Source: CAD feature listing. Evaluate the final solid. Frame: model axes, mm. A direction names the side the tool comes from. Round coordinates to 2 decimals unless told otherwise and drop trailing zeros. Write each loop counter-clockwise with the first axis right and the second up, starting at its lowest first coordinate (ties: lowest second). Pieces come first, ordered by that corner, then holes. Notation, with made-up numbers: M -15,-15.5 L 34,-15.5 A33 ccw 34,15.5 Z; hole C 28,26 d5. An arc over 180 degrees is marked long. Answer in a Markdown table with one row per item.
from build123d import *

# Parameters (mm, degrees)
SKETCH1_R           = 13.4
BOSS_EXTRUDE1_DEPTH = 56
SKETCH2_W           = 100
SKETCH2_H           = 60
BOSS_EXTRUDE2_DEPTH = 4
SKETCH3_R           = 13.4
CUT_EXTRUDE1_DEPTH  = 25.2
SKETCH4_W           = 25.2
SKETCH4_H           = 25.2
CUT_EXTRUDE2_DEPTH  = 51.2


with BuildPart() as part:
    # Sketch1 → Boss-Extrude1 (new body)
    with BuildSketch(Plane(origin=(0, 0, 0), x_dir=(1, 0, 0), z_dir=(0, 1, 0))):
        Polygon((-65.2, -11.320132013), (-65.2, 44.679867987), (0, 44.679867987), (0, 48.679867987), (-100, 48.679867987), (-100, -11.320132013), align=None)
        with Locations(Location((-82.6, 31.279867987, 0), (0, 0, 270))):
            Circle(SKETCH1_R, mode=Mode.SUBTRACT)
    extrude(amount=BOSS_EXTRUDE1_DEPTH)

    # Sketch2 → Boss-Extrude2 (add)
    with BuildSketch(Plane(origin=(0, 0, 0), x_dir=(1, 0, 0), z_dir=(0, 1, 0))):
        with Locations((-50, 18.679867987)):
            Rectangle(SKETCH2_W, SKETCH2_H)
    extrude(amount=-BOSS_EXTRUDE2_DEPTH)

    # Sketch3 → Cut-Extrude1 (cut)
    with BuildSketch(Plane.XY.offset(11.320132013)):
        with Locations((-82.6, 13.4)):
            Circle(SKETCH3_R)
    extrude(amount=-CUT_EXTRUDE1_DEPTH, mode=Mode.SUBTRACT)

    # Sketch4 → Cut-Extrude2 (cut)
    with BuildSketch(Plane.ZY.offset(100)):
        with Locations((-1.279867987, 43.4)):
            Rectangle(SKETCH4_W, SKETCH4_H)
    extrude(amount=-CUT_EXTRUDE2_DEPTH, mode=Mode.SUBTRACT)


solid = part.part
Q1. Access query for faces 4 (the cylindrical face through (-69.819, 17.425, -1.103)), 5 (the flat face through (-83, 30.8, -1)), 6 (the flat face through (-65.2, 21, -23)). Directions: +Z, -Z, +X, -X, +Y, -Y. A direction counts if a zero-diameter tool reaches every point of the face in a straight line with its end or side. Return the directions, or none.
Solutions:
| item | result |
|---|---|
| face 4 | +Z |
| face 5 | +Z, +X, -X, +Y |
| face 6 | +Z, +X, +Y |
Q2. Section A-A (y = 13.4). Return loops of the section in (x, z), and give its area (3 significant figures).
Solutions:
| item | result |
|---|---|
| outline | M -100,-48.68 L 0,-48.68 L 0,-44.68 L -65.2,-44.68 L -65.2,11.32 L -69.2,11.32 L -69.2,-13.88 L -96,-13.88 L -96,11.32 L -100,11.32 Z; hole C -82.6,-31.28 d26.8 |
| area | 1,110 mm2 |
Q3. Contact query for flat-ended pins moving along their axis: pin 1 Ø2 at (x, y) = (-50, 37) entering from +Z; pin 2 Ø12.5 at (x, y) = (-84, 49) entering from +Z; pin 3 Ø13.5 at (x, z) = (-84, -28) entering from +Y. Output: stop coordinate, or through.
Solutions:
| item | result |
|---|---|
| pin 1 | stops at z = -44.68 |
| pin 2 | stops at z = -13.88 |
| pin 3 | stops at y = 0 |
Q4. Section C-C (x = -82.6). Return loops of the section in (y, z).
Solutions:
| item | result |
|---|---|
| outline | M -4,-48.68 L 56,-48.68 L 56,-44.68 L 0,-44.68 L 0,-17.88 L 56,-17.88 L 56,-13.88 L 30.8,-13.88 L 30.8,11.32 L 26.8,11.32 L 26.8,-13.88 L 0,-13.88 L 0,11.32 L -4,11.32 Z |
Q5. Material intervals for probe 1 along Z at (x, y) = (-82, 37); probe 2 along Y at (x, z) = (-82, 6); probe 3 along X at (y, z) = (13, 0), sorted ascending.
Solutions:
| item | result |
|---|---|
| probe 1 | z = -48.68 to -44.67, -17.89 to -13.88 |
| probe 2 | y = -4 to 0.01, 26.79 to 30.8 |
| probe 3 | x = -100 to -95.99, -69.21 to -65.2 |
Q6. Pull-direction query (Y, two-part tool) for faces 1 (the flat face through (-83, 14, -13.88)), 2 (the flat face through (-83, 0, -31)), 3 (the flat face through (-83, 43, -13.88)); classes: pulls with the +Y half, pulls with the -Y half, needs draft (parallel to the pull), parting line crosses it, or undercut.
Solutions:
| item | result |
|---|---|
| face 1 | undercut |
| face 2 | pulls with the +Y half |
| face 3 | needs draft |
Q7. Section B-B (z = -9). Return loops of the section in (x, y), and give its area (3 significant figures).
Solutions:
| item | result |
|---|---|
| outline | M -100,-4 L 0,-4 L 0,0 L -65.2,0 L -65.2,30.8 L -100,30.8 Z; hole C -82.6,13.4 d26.8 |
| area | 908 mm2 |
Q8. Section D-D (y = 47). Return loops of the section in (x, z).
Solutions:
| item | result |
|---|---|
| outline | M -100,-48.68 L 0,-48.68 L 0,-44.68 L -65.2,-44.68 L -65.2,-13.88 L -100,-13.88 Z; hole C -82.6,-31.28 d26.8 |
